from build123d import *

# Parameters (mm, degrees)
F0_W      = 1500
F0_H      = 280
F1_DEPTH  = 210
F2_W      = 1500
F2_H      = 280
F2_W_2    = 1494
F2_H_2    = 274
F3_DEPTH  = 100
F5_DEPTH  = 1500
F6_R      = 75
F7_DEPTH  = 5
F8_R      = 75
F9_DEPTH  = 5
F11_DEPTH = 3
F13_DEPTH = 3


with BuildPart() as f1:
    # F0 (on Front) → F1 (new body)
    with BuildSketch(Plane.XZ):
        Rectangle(F0_W, F0_H)
    extrude(amount=-F1_DEPTH)

    # F2 (on face) → F3 (join)
    with BuildSketch(Plane.XZ):
        Rectangle(F2_W, F2_H)
        Rectangle(F2_W_2, F2_H_2, mode=Mode.SUBTRACT)
    extrude(amount=F3_DEPTH)

    # F4 (on face) → F5 (join)
    with BuildSketch(Plane.YZ.offset(750)):
        Polygon((-866.044443, 782.78761), (-100, 140), (-95.058616, 140), (-863.438088, 784.746932), (-863.438088, 787.488366), (-866.044443, 787.488366), align=None)
        Polygon((-95.058616, -140), (-100, -140), (-866.044443, -782.78761), (-866.044443, -787.488366), (-863.438088, -787.488366), (-863.438088, -784.746932), align=None)
    extrude(amount=-F5_DEPTH)

    # F6 (on face) → F7 (join)
    with BuildSketch(Plane.YZ.offset(750)):
        with Locations((57.470692, 0)):
            Circle(F6_R)
    extrude(amount=F7_DEPTH)

    # F8 (on face) → F9 (join)
    with BuildSketch(Plane(origin=(-750, 0, 0), x_dir=(0, -1, 0), z_dir=(-1, 0, 0))):
        with Locations((-57.470692, 0)):
            Circle(F8_R)
    extrude(amount=F9_DEPTH)

    # F10 (on face) → F11 (join)
    with BuildSketch(Plane(origin=(-750, 0, 0), x_dir=(0, -1, 0), z_dir=(-1, 0, 0))):
        Polygon((866.044443, 787.488366), (863.438088, 787.488366), (863.438088, 784.746932), (95.058616, 140), (100, 140), (100, -140), (95.058616, -140), (863.438088, -784.746932), (863.438088, -787.488366), (866.044443, -787.488366), (866.044443, -782.78761), (866.044443, 782.78761), align=None)
    extrude(amount=-F11_DEPTH)

    # F12 (on face) → F13 (join)
    with BuildSketch(Plane.YZ.offset(750)):
        Polygon((-866.044443, -782.78761), (-866.044443, -787.488366), (-863.438088, -787.488366), (-863.438088, -784.746932), (-95.058616, -140), (-100, -140), (-100, 140), (-95.058616, 140), (-863.438088, 784.746932), (-863.438088, 787.488366), (-866.044443, 787.488366), (-866.044443, 782.78761), align=None)
    extrude(amount=-F13_DEPTH)


solid = f1.part
Geometry check sheet. Reference: the model listing, model coordinates, mm. A direction names the side the tool comes from. Round coordinates to 2 decimals unless told otherwise and drop trailing zeros. Loops run counter-clockwise (first coordinate to the right, second up) from the corner with the lowest first, then second, coordinate; pieces in that order, holes last. Notation, with made-up numbers: (15.5, 47.5) - (55.5, 47.5) arc R21 cw to (55.5, 76.5) - close; hole circle Ø6 at (36, 51.25). An arc over 180 degrees is marked (long way). One line per question, with ' | ' between items. Start each with the question number.
1. Cross-section at A-A on x = -224. Record the cut outline in (y, z), then the cut area to 3 significant figures.
2. Depth check by flat-ended pin: pin 1 (1.4 mm diameter, centred on x = -121, z = -786.5, fed in from +Y); pin 2 (3.5 mm diameter, centred on x = -82.5, z = -138.5, fed in from -Y); pin 3 (6 mm diameter, centred on x = 127, y = -322.5, fed in from +Z). Enter the tip coordinate at first touch or a pass-through.
3. Tool access check on faces 1 (the face through (-10, 60, 140)), 2 (the face through (-10, -49, -137)), 3 (the face through (752.465, -17.457, 3.298)). Record the directions out of +Z, -Z, +X, -X, +Y, -Y that give a thin tool (end or side, any length) a straight path to the whole face; none if there is none.
4. Cross-section at B-B on z = 0. Record the cut outline in (x, y), then the cut area to 3 significant figures.
5. Scan lines: line 1 (X direction, y = -665, z = -202.5); line 2 (Z direction, x = -132, y = 126); line 3 (Z direction, x = -193, y = -557). Record each from-to range of solid material in increasing order. Write a range as [from, to].
6. Draft check along Z on faces 4 (the face through (747, -535, 11)), 5 (the face through (10.5, -473.87, 457.86)), 6 (the face through (-10, -49, 137)), 7 (the face through (-755, 59, 1)). Enter one of: released by +Z, released by -Z, zero draft, split by the parting line, or undercut.
7. Cross-section at D-D on z = -507. Record the cut outline in (x, y).
8. Cross-section at C-C on y = -645.5. Record the cut outline in (x, z), then the cut area to 3 significant figures.
Taken from the geometry:
1) outline: (-866.04, -787.49) - (-863.44, -787.49) - (-863.44, -784.75) - (-95.06, -140) - (210, -140) - (210, 140) - (-95.06, 140) - (-863.44, 784.75) - (-863.44, 787.49) - (-866.04, 787.49) - (-866.04, 782.79) - (-100, 140) - (-100, 137) - (0, 137) - (0, -137) - (-100, -137) - (-100, -140) - (-866.04, -782.79) - close | area: 65,800 mm²
2) pin 1: y = -863.44 | pin 2: y = -100.3 | pin 3: z = 333.36
3) face 1: +Z, +X, -X, +Y | face 2: -Y | face 3: +X
4) outline: (-755, -17.53) - (-750, -17.53) - (-750, -866.04) - (-747, -866.04) - (-747, 0) - (747, 0) - (747, -866.04) - (750, -866.04) - (750, -17.53) - (755, -17.53) - (755, 132.47) - (750, 132.47) - (750, 210) - (-750, 210) - (-750, 132.47) - (-755, 132.47) - close | area: 322,000 mm²
5) line 1: [-750, -747], [747, 750] | line 2: [-140, 140] | line 3: [-527.61, -523.47], [523.47, 527.61]
6) face 4: undercut | face 5: released by +Z | face 6: undercut | face 7: zero draft
7) outline: (-750, -866.04) - (-747, -866.04) - (-747, -537.37) - (747, -537.37) - (747, -866.04) - (750, -866.04) - (750, -532.43) - (-750, -532.43) - close
8) outline: (-750, -601.88) - (750, -601.88) - (750, 601.88) - (-750, 601.88) - close; hole (-747, -597.73) - (747, -597.73) - (747, 597.73) - (-747, 597.73) - close | area: 19,600 mm²
